Can you work these out from the drawing? Everything is in mm from the part's minimum corner. Give positions to 0.01 mm unless a question says otherwise; leave off trailing zeros. Order: outer loops, then holes, each group sorted by start corner. A loop starts at its lowest first (then second) coordinate and runs counter-clockwise, first axis right, second up. Notation, with made-up numbers: (11.25, 81.5) - (54.25, 81.5) arc R13 cw to (54.25, 96.5) - close; hole circle Ø7 at (54.5, 25.5). An arc over 180 degrees is marked (long way). Write each question's results on one line, items separated by ' | '. Start each with the question number.
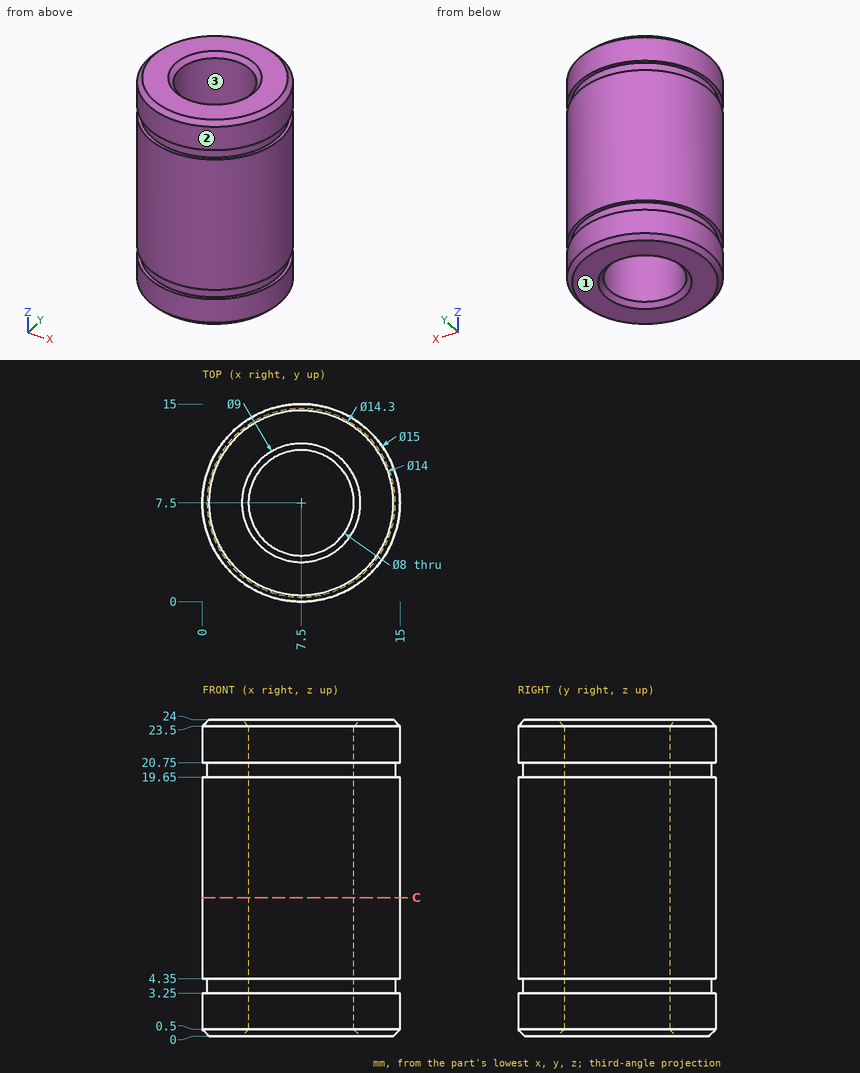
Q1. Will these pins go through, and if not, where does the flat tip stop? P1, Ø7.5, axis at x = 4, y = 6.5, coming from the +Z side; P2, Ø4.5, axis at x = 6, y = 6.5, coming from the -Z side; P3, Ø4, axis at y = 3, z = 6, coming from the +X side; P4, Ø1, axis at x = 11.5, z = 5.5, coming from the +Y side.
Q2. If we section it at C-C (z = 10.5): Please give me the cut outline in (x, y), plus the area to 3 significant figures.
Q3. Thinking about a two-plate mould opening in Y: for the marked faces 1, 2 and 3, which applies, released by +Y, released by -Y, zero draft, split by the parting line, or undercut?
Q4. If I drill on probe 1 along Y at (x, z) = (7.5, 13); probe 2 along Z at (x, y) = (14.75, 6); probe 3 along Y at (x, z) = (8.75, 6), over which ranges is the centre line in solid material (lowest first)? Write a range as from..to.
Findings below:
1) P1: stops at z = 24 | P2: stops at z = 0.45 | P3: stops at x = 14.57 | P4: stops at y = 14.13
2) outline: circle Ø15 at (7.5, 7.5); hole circle Ø8 at (7.5, 7.5) | area: 126 mm2
3) face 1: zero draft | face 2: split by the parting line | face 3: undercut
4) probe 1: y = 0..3.5, 11.5..15 | probe 2: z = 0.4..3.25, 4.35..19.65, 20.75..23.6 | probe 3: y = 0.1..3.7, 11.3..14.9
